from build123d import *

# Parameters (mm, degrees)
SKETCH1_R           = 6
BOSS_EXTRUDE1_DEPTH = 2.535


with BuildPart() as part:
    # Sketch1 → Boss-Extrude1 (new, symmetric)
    # profile 1 of 2: a face of its own
    with BuildSketch(Plane(origin=(0, 0, 0), x_dir=(0, 1, 0), z_dir=(0, 0, 1))):
        with BuildLine():
            ThreePointArc((11.5, 0), (0, 11.5), (-11.5, 0))
            ThreePointArc((-11.5, 0), (0, -11.5), (11.5, 0))
        make_face()
        with Locations(Location((0, 0, 0), (0, 0, 270))):
            Circle(SKETCH1_R, mode=Mode.SUBTRACT)
    # profile 2 of 2: a face of its own
    with BuildSketch(Plane(origin=(0, 0, 0), x_dir=(0, 1, 0), z_dir=(0, 0, 1))):
        with BuildLine():
            ThreePointArc((11.5, 0), (0, -11.5), (-11.5, 0))
            Line((-11.5, 0), (-11.5, -16))
            Line((-11.5, -16), (11.5, -18.040557186))
            Line((11.5, -18.040557186), (11.5, 0))
        make_face()
    extrude(amount=BOSS_EXTRUDE1_DEPTH, both=True)


solid = part.part
Could you check a few things on this model? Use its own coordinates, in mm. Give positions to 0.01 mm unless a question says otherwise; leave off trailing zeros. Order: outer loops, then holes, each group sorted by start corner. A loop starts at its lowest first (then second) coordinate and runs counter-clockwise, first axis right, second up.
1. Suppose I cut it at C-C (x = -1.75). Write out the boundary of the cut face in (y, z) (3 decimals), plus the area to 3 significant figures.
Answers below:
outline: (-11.366, -2.535) - (-5.739, -2.535) - (-5.739, 2.535) - (-11.366, 2.535) - close; (5.739, -2.535) - (11.366, -2.535) - (11.366, 2.535) - (5.739, 2.535) - close
area: 57.1 mm2
2. I need wall thicknesses on L1, parallel to Y at x = 0, z = -1.6; L2, parallel to X at y = -1.5, z = -0.3; L3, parallel to Y at x = -5, z = -0.9. Which ranges of each line are inside material? Lowest first, please.
Answers below:
L1: y = -11.5 to -6, 6 to 11.5
L2: x = -11.4 to -5.81, 5.81 to 16.89
L3: y = -10.36 to -3.32, 3.32 to 10.36
3. For pin 1 (11 mm diameter, centred on x = 0, y = 0, fed in from +Z), with a flat end and sliding along its axis, tell me the tip position at first contact or that it passes through.
Answers below:
pin 1: passes through
4. Suppose I cut it at D-D (y = 7.5). Write out the boundary of the cut face in (x, z) (3 decimals).
Answers below:
outline: (-8.718, -2.535) - (17.686, -2.535) - (17.686, 2.535) - (-8.718, 2.535) - close
5. Suppose I cut it at B-B (z = -2.1). Write out the boundary of the cut face in (x, y), plus the area to 3 significant figures.
Answers below:
outline: (0, -11.5) - (16, -11.5) - (18.04, 11.5) - (0, 11.5) arc R11.5 ccw to start; hole circle Ø12 at (0, 0)
area: 486 mm2
6. Suppose I cut it at A-A (y = 4.75). Write out the boundary of the cut face in (x, z) (3 decimals).
Answers below:
outline: (-10.473, -2.535) - (-3.666, -2.535) - (-3.666, 2.535) - (-10.473, 2.535) - close; (3.666, -2.535) - (17.442, -2.535) - (17.442, 2.535) - (3.666, 2.535) - close
